```python
from build123d import *

# Parameters (mm, degrees)
SKETCH_W        = 80
SKETCH_H        = 260
PAD_DEPTH       = 3
SKETCH004_R     = 2.25
HOLE002_DEPTH   = 3.001
SKETCH006_R     = 1.5
SKETCH006_W     = 36
SKETCH006_H     = 3
SKETCH006_W_2   = 3
SKETCH006_H_2   = 16
POCKET_DEPTH    = 3.001
SKETCH012_R     = 8.25
POCKET003_DEPTH = 3.001


with BuildPart() as part:
    # Sketch → Pad (new body)
    with BuildSketch(Plane.XY):
        Rectangle(SKETCH_W, SKETCH_H)
    extrude(amount=PAD_DEPTH)

    # Sketch004 (on Face6 of Pad) → Hole002 (cut, through all)
    with BuildSketch(Plane.XY.offset(3)):
        with Locations((-25, -120)):
            Circle(SKETCH004_R)
        with Locations((-25, 120)):
            Circle(SKETCH004_R)
        with Locations((30, 0)):
            Circle(SKETCH004_R)
        with Locations((30, -95)):
            Circle(SKETCH004_R)
        with Locations((30, 95)):
            Circle(SKETCH004_R)
    extrude(amount=-HOLE002_DEPTH, mode=Mode.SUBTRACT)

    # Sketch006 (on Face5 of Hole002) → Pocket (cut, through all)
    with BuildSketch(Plane.XY.offset(3)):
        with Locations((-28.5, 13.5)):
            Circle(SKETCH006_R)
        with Locations((13.5, 13.5)):
            Circle(SKETCH006_R)
        with Locations((-11.5, -11)):
            Circle(SKETCH006_R)
        with Locations((-7.5, 13.5)):
            Rectangle(SKETCH006_W, SKETCH006_H)
        with Locations((-11.5, 0)):
            Rectangle(SKETCH006_W_2, SKETCH006_H_2)
    extrude(amount=-POCKET_DEPTH, mode=Mode.SUBTRACT)

    # Sketch012 (on Face4 of Pocket) → Pocket003 (cut, through all)
    with BuildSketch(Plane(origin=(0, 0, 0), x_dir=(1, 0, 0), z_dir=(0, 0, -1))):
        with Locations((-15, 75)):
            Circle(SKETCH012_R)
    extrude(amount=-POCKET003_DEPTH, mode=Mode.SUBTRACT)


with BuildPart() as part_1:
    # Body placement: moved
    add(part.part.moved(Location((-170, 141, 81))))


solid = part_1.part
```
Here's how the part is built. I have some questions about the finished solid (model axes, mm). Round coordinates to 2 decimals unless told otherwise and drop trailing zeros. Loops run counter-clockwise (first coordinate to the right, second up) from the corner with the lowest first, then second, coordinate; pieces in that order, holes last.
1. Suppose I cut it at A-A, the plane y = 46. Please give me the cut outline in (x, z), and give its area (4 significant figures).
Answers:
outline: (-210, 81) - (-142.25, 81) - (-142.25, 84) - (-210, 84) - close; (-137.75, 81) - (-130, 81) - (-130, 84) - (-137.75, 84) - close
area: 226.5 mm2
2. Suppose I cut it at B-B, the plane z = 83.5. Give the number of separate pieces and of enclosed holes in the cut face, and give its area (3 significant figures).
Answers:
separate pieces: 1
enclosed holes: 11
area: 20,300 mm2
3. Thinking about a two-plate mould opening in Y: for faces 1 (the face through (-171, 143, 84)), 2 (the face through (-180.565, 59.044, 82.479)), which applies, released by +Y, released by -Y, zero draft, split by the parting line, or undercut?
Answers:
face 1: zero draft
face 2: undercut
4. Will these pins go through, and if not, where does the flat tip stop? pin 1 (5 mm diameter, centred on x = -181.5, y = 130, fed in from +Z); pin 2 (2.5 mm diameter, centred on x = -156.5, y = 154.5, fed in from +Z).
Answers:
pin 1: stops at z = 84
pin 2: passes through
5. If I drill on probe 1 along Y at (x, z) = (-185, 83.15); probe 2 along Y at (x, z) = (-195, 81.85); probe 3 along Y at (x, z) = (-140, 81.85), over which ranges is the centre line in solid material (lowest first)?
Answers:
probe 1: y = 11 to 57.75, 74.25 to 153, 156 to 271
probe 2: y = 11 to 18.75, 23.25 to 153, 156 to 258.75, 263.25 to 271
probe 3: y = 11 to 43.75, 48.25 to 138.75, 143.25 to 233.75, 238.25 to 271
